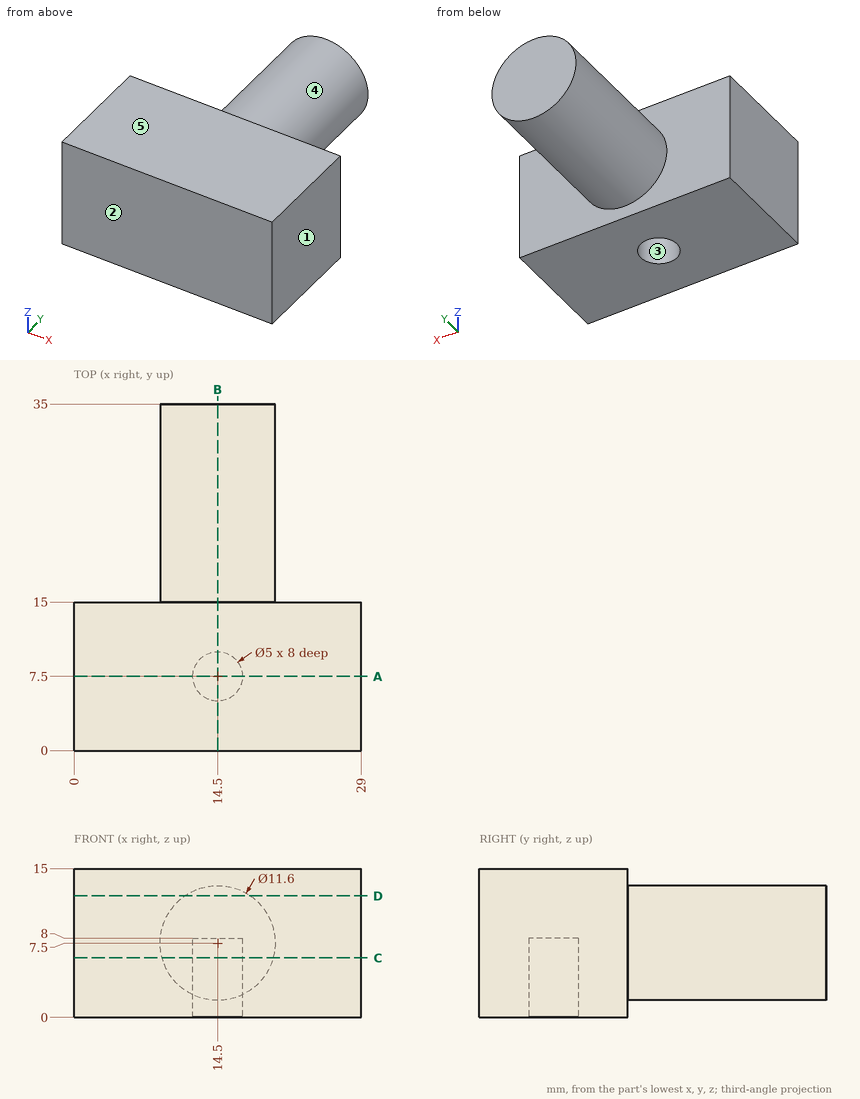
Source: three-view drawing plus pictorial views. Frame: mm from the lowest corner of the part. A direction names the side the tool comes from. Round coordinates to 2 decimals unless told otherwise and drop trailing zeros. Loops run counter-clockwise (first coordinate to the right, second up) from the corner with the lowest first, then second, coordinate; pieces in that order, holes last. Notation, with made-up numbers: M 30,39 L 35,39 A21 ccw 35,70 Z; hole C -24.75,14 d8. An arc over 180 degrees is marked long. Answer as CSV lines item,"result".
Q1. Line query: line 1 along Y through (x, z) = (14.5, 6); line 2 along Z through (x, y) = (14.25, 8.5); line 3 along Z through (x, y) = (14.75, 16.5). Output: solid intervals per line, ascending.
Verdict:
line 1,"y = 0 to 5, 10 to 35"
line 2,"z = 8 to 15"
line 3,"z = 1.71 to 13.29"
Q2. Cut plane B-B (x = 14.5). Return the cut outline in (y, z), plus the area to 3 significant figures.
Verdict:
outline,"M 0,0 L 5,0 L 5,8 L 10,8 L 10,0 L 15,0 L 15,1.7 L 35,1.7 L 35,13.3 L 15,13.3 L 15,15 L 0,15 Z"
area,"417 mm^2"
Q3. Reachability of the marked faces 4 and 5 from +Z, -Z, +X, -X, +Y, -Y: full face, straight path, thin tool, end or side. Return the list, or none.
Verdict:
face 4,"+Y"
face 5,"+Z, +X, -X, +Y, -Y"
Q4. Cut plane C-C (z = 6). Return the cut outline in (x, y).
Verdict:
outline,"M 0,0 L 29,0 L 29,15 L 20.1,15 L 20.1,35 L 8.9,35 L 8.9,15 L 0,15 Z; hole C 14.5,7.5 d5"
Q5. Cut plane A-A (y = 7.5). Return the cut outline in (x, z), plus the area to 3 significant figures.
Verdict:
outline,"M 0,0 L 12,0 L 12,8 L 17,8 L 17,0 L 29,0 L 29,15 L 0,15 Z"
area,"395 mm^2"
Q6. Pull-direction query (X, two-part tool) for the marked faces 1, 2 and 3; classes: +X half, -X half, draft (parallel to the pull), parting line (faces both ways), or undercut.
Verdict:
face 1,"+X half"
face 2,"draft"
face 3,"undercut"
Q7. Cut plane D-D (z = 12.25). Return the cut outline in (x, y), plus the area to 3 significant figures.
Verdict:
outline,"M 0,0 L 29,0 L 29,15 L 17.83,15 L 17.83,35 L 11.17,35 L 11.17,15 L 0,15 Z"
area,"568 mm^2"
Q8. Contact query for flat-ended pins moving along their axis: pin 1 (1.5 mm diameter, centred on x = 15, y = 6.5, fed in from -Z); pin 2 (1 mm diameter, centred on x = 22, z = 5.5, fed in from +Y); pin 3 (4 mm diameter, centred on x = 6, y = 30.5, fed in from +Z); pin 4 (2 mm diameter, centred on x = 13.5, y = 23, fed in from -Z). Output: stop coordinate, or through.
Verdict:
pin 1,"stops at z = 8"
pin 2,"stops at y = 15"
pin 3,"passes through"
pin 4,"stops at z = 1.7"
